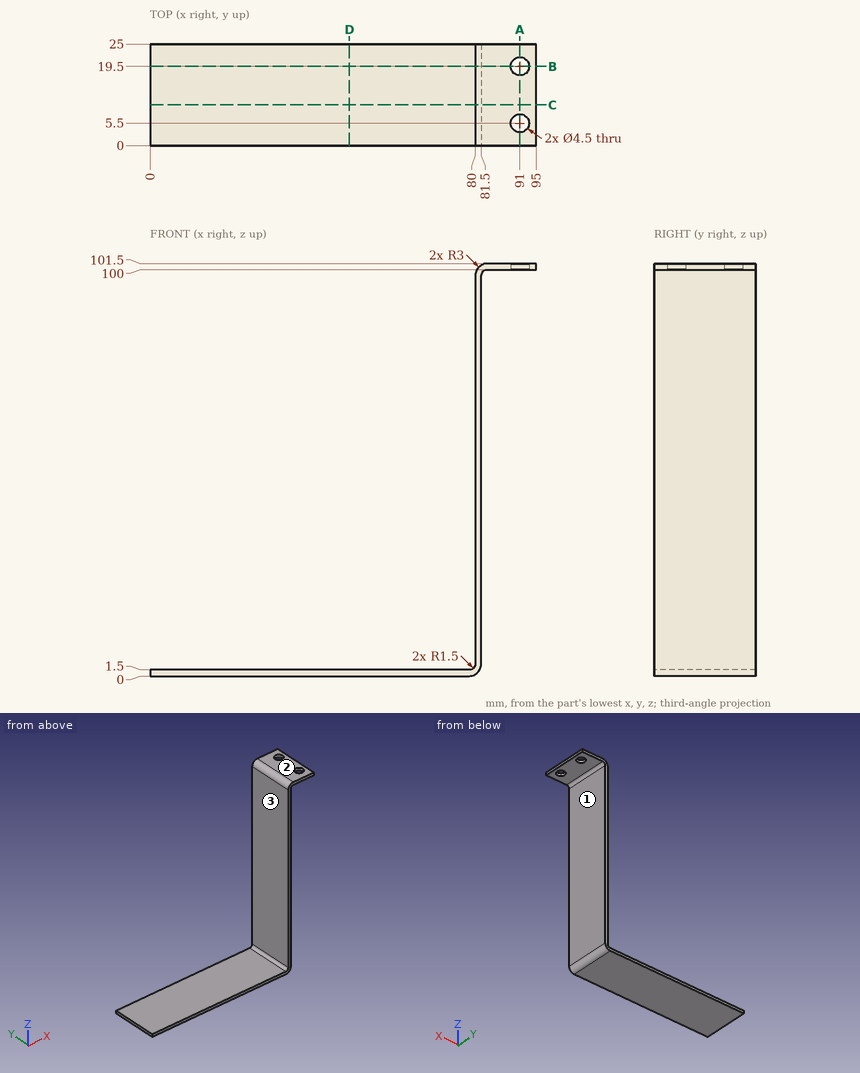
Part print with two shaded views. Sizes in mm from the minimum x, y, z corner. A direction names the side the tool comes from. Round coordinates to 2 decimals unless told otherwise and drop trailing zeros. Order: outer loops, then holes, each group sorted by start corner. A loop starts at its lowest first (then second) coordinate and runs counter-clockwise, first axis right, second up. Notation, with made-up numbers: (80, 60) -> (95, 60) arc R29 cw to (95, 85) -> close; hole circle Ø6 at (71.25, -34). An arc over 180 degrees is marked (long way). Write each question's results on one line, items separated by ' | '.
1. Wall check: line 1 along Y through (x, z) = (91, 100.95); line 2 along Z through (x, y) = (84, 19); line 3 along Z through (x, y) = (60.5, 10.5). Give the ranges that are in metal, low to high. Write a range as [from, to].
Findings below:
line 1: y = [0, 3.25], [7.75, 17.25], [21.75, 25] | line 2: z = [100, 101.5] | line 3: z = [0, 1.5]
2. 3-axis set-ups, long thin cutter, end or side, ignore diameter. For the marked faces 1, 2 and 3: which of +Z, -Z, +X, -X, +Y, -Y reach the whole face in a straight line?
Findings below:
face 1: -Z, +X, +Y, -Y | face 2: +Z, +X, -X, +Y, -Y | face 3: +Z, -X, +Y, -Y
3. Cut at D-D (x = 49). Give the cut face in (y, z), plus the area to 3 significant figures.
Findings below:
outline: (0, 0) -> (25, 0) -> (25, 1.5) -> (0, 1.5) -> close | area: 37.5 mm²
4. Cut at C-C (y = 10). Give the cut face in (x, z).
Findings below:
outline: (0, 0) -> (78.5, 0) arc R3 ccw to (81.5, 3) -> (81.5, 98.5) arc R1.5 cw to (83, 100) -> (95, 100) -> (95, 101.5) -> (83, 101.5) arc R3 ccw to (80, 98.5) -> (80, 3) arc R1.5 cw to (78.5, 1.5) -> (0, 1.5) -> close
5. Cut at A-A (x = 91). Give the cut face in (y, z).
Findings below:
outline: (0, 100) -> (3.25, 100) -> (3.25, 101.5) -> (0, 101.5) -> close; (7.75, 100) -> (17.25, 100) -> (17.25, 101.5) -> (7.75, 101.5) -> close; (21.75, 100) -> (25, 100) -> (25, 101.5) -> (21.75, 101.5) -> close
6. Flat gauge pins, fed straight in: P1, Ø12, axis at x = 43.5, y = 5, coming from the +Z side; P2, Ø9.5, axis at x = 89, y = 8.5, coming from the -Z side; P3, Ø7.5, axis at y = 6.5, z = 64.5, coming from the +X side. Where does each tip first touch, or does it go through?
Findings below:
P1: stops at z = 1.5 | P2: stops at z = 100 | P3: stops at x = 81.5
7. Cut at B-B (y = 19.5). Give the cut face in (x, z), plus the area to 3 significant figures.
Findings below:
outline: (0, 0) -> (78.5, 0) arc R3 ccw to (81.5, 3) -> (81.5, 98.5) arc R1.5 cw to (83, 100) -> (88.75, 100) -> (88.75, 101.5) -> (83, 101.5) arc R3 ccw to (80, 98.5) -> (80, 3) arc R1.5 cw to (78.5, 1.5) -> (0, 1.5) -> close; (93.25, 100) -> (95, 100) -> (95, 101.5) -> (93.25, 101.5) -> close | area: 283 mm²
